from build123d import *

# Parameters (mm, degrees)
PAD_DEPTH       = 40
SKETCH001_W     = 20.2
SKETCH001_H     = 5
SKETCH001_W_2   = 5
SKETCH001_H_2   = 20.2
POCKET_DEPTH    = 5
SKETCH002_R     = 2.75
POCKET001_DEPTH = 5.001
POCKET002_DEPTH = 5.001


with BuildPart() as part:
    # Sketch → Pad (new body)
    with BuildSketch(Plane.XY):
        Polygon((0, 0), (-35, 0), (-35, -5), (-5, -5), (-5, -35), (0, -35), align=None)
    extrude(amount=PAD_DEPTH)

    # Sketch001 (on Face8 of Pad) → Pocket (cut)
    with BuildSketch(Plane.XY.offset(40)):
        with Locations((-20, -2.5)):
            Rectangle(SKETCH001_W, SKETCH001_H)
        with Locations((-2.5, -20)):
            Rectangle(SKETCH001_W_2, SKETCH001_H_2)
    extrude(amount=-POCKET_DEPTH, mode=Mode.SUBTRACT)

    # Sketch002 (on Face10 of Pocket) → Pocket001 (cut, through all)
    with BuildSketch(Plane.XZ.offset(5)):
        with Locations((-20, 17.5)):
            Circle(SKETCH002_R)
    extrude(amount=-POCKET001_DEPTH, mode=Mode.SUBTRACT)

    # Sketch003 (on Face12 of Pocket001) → Pocket002 (cut, through all)
    with BuildSketch(Plane(origin=(-5, 0, 0), x_dir=(0, -1, 0), z_dir=(-1, 0, 0))):
        with BuildLine():
            Line((17.25, 0), (22.75, 0))
            Line((22.75, 0), (22.75, 17.5))
            ThreePointArc((22.75, 17.5), (20, 20.25), (17.25, 17.5))
            Line((17.25, 17.5), (17.25, 0))
        make_face()
    extrude(amount=-POCKET002_DEPTH, mode=Mode.SUBTRACT)


solid = part.part
Geometry check sheet. Reference: the model listing, model coordinates, mm. A direction names the side the tool comes from. Give positions to 0.01 mm unless a question says otherwise; leave off trailing zeros. Loops run counter-clockwise (first coordinate to the right, second up) from the corner with the lowest first, then second, coordinate; pieces in that order, holes last. Notation, with made-up numbers: M 66.5,-37.5 L 71.5,-37.5 A12 ccw 71.5,-21.5 Z; hole C -38.75,-13.5 d9. An arc over 180 degrees is marked long. Answer as a JSON object with one key per item and string values. Group by question number.
Item 1: Sectioned sample at A-A on z = 6. Record the boundary of the cut face in (x, y).
Item 2: Sectioned sample at C-C on z = 24.5. Record the boundary of the cut face in (x, y).
Item 3: Material ranges on L1, parallel to Z at x = -20, y = -2; L2, parallel to Y at x = -4, z = 6.5; L3, parallel to Y at x = -7, z = 24, recorded low to high.
Item 4: Mould release check, pull along Z, two halves, no side actions. Record for faces 5 (the flat face through (-3, -33, 40)), 6 (the flat face through (-3, -22.75, 9)), 7 (the cylindrical face through (-22.747, -2.535, 17.621)): pulls with the +Z half, pulls with the -Z half, needs draft (parallel to the pull), parting line crosses it, or undercut.
Item 5: Gauge pin test, flat ends, axial feed: pin 1 (5 mm diameter, centred on x = -27.5, z = 34.5, fed in from -Y); pin 2 (2 mm diameter, centred on y = -18.5, z = 26, fed in from -X); pin 3 (4 mm diameter, centred on x = -20, y = -2, fed in from +Z); pin 4 (2 mm diameter, centred on y = -21.5, z = 12, fed in from -X). Record the tip position at first contact, or that the pin passes through.
Item 6: Sectioned sample at B-B on x = -20. Record the boundary of the cut face in (y, z), plus the area to 4 significant figures.
Item 7: Sectioned sample at D-D on y = -24.5. Record the boundary of the cut face in (x, z), plus the area to 3 significant figures.
Item 8: Access from +Z, -Z, +X, -X, +Y, -Y to the whole of each face (thin tool, end or side, straight path). Record for faces 1 (the flat face through (-30.1, -3, 38)), 2 (the flat face through (-24, -5, 20)), 3 (the flat face through (-3, -20, 35)), 4 (the flat face through (-3, -17.25, 9)).
Findings below:
{
 "1": {"outline": "M -35,-5 L -5,-5 L -5,-17.25 L 0,-17.25 L 0,0 L -35,0 Z; M -5,-35 L 0,-35 L 0,-22.75 L -5,-22.75 Z"},
 "2": {"outline": "M -35,-5 L -5,-5 L -5,-35 L 0,-35 L 0,0 L -35,0 Z"},
 "3": {"L1": "0 to 14.75, 20.25 to 35", "L2": "-35 to -22.75, -17.25 to 0", "L3": "-5 to 0"},
 "4": {"face 5": "pulls with the +Z half", "face 6": "needs draft", "face 7": "undercut"},
 "5": {"pin 1": "y = -5", "pin 2": "x = -5", "pin 3": "z = 35", "pin 4": "through"},
 "6": {"outline": "M -5,0 L 0,0 L 0,14.75 L -5,14.75 Z; M -5,20.25 L 0,20.25 L 0,35 L -5,35 Z", "area": "147.5 mm2"},
 "7": {"outline": "M -5,0 L 0,0 L 0,35 L -5,35 Z", "area": "175 mm2"},
 "8": {"face 1": "+Z, +Y, -Y", "face 2": "+Z, -Z, -X, -Y", "face 3": "+Z, +X, -X", "face 4": "-Z, +X, -X"}
}
